Read the model definition and answer for the solid it produces. Units are mm, in the model's axes. A direction names the side the tool comes from. Round coordinates to 2 decimals unless told otherwise and drop trailing zeros. Order: outer loops, then holes, each group sorted by start corner. A loop starts at its lowest first (then second) coordinate and runs counter-clockwise, first axis right, second up. Notation, with made-up numbers: (41, 13) - (54, 13) arc R31 cw to (54, 42) - close; hole circle Ø9 at (-12, -7). An arc over 180 degrees is marked (long way). Answer as a JSON object with one key per item and string values. Group by question number.
Q1. A cutting plane is placed at A-A on x = -3.5. Determine the outline of the cut face in (y, z), and give its area (3 significant figures).
Q2. A cutting plane is placed at D-D on z = -12. Determine the outline of the cut face in (x, y), and give its area (3 significant figures).
Q3. A cutting plane is placed at B-B on z = -65. Determine the outline of the cut face in (x, y).
Q4. The mould has two halves that part along Z. Classify faces 1 (the flat face through (40, 11, -15)), 2 (the cylindrical face through (42.39, 4.27, -66.67)), 3 (the flat face through (10, 63, 24)): pulls with the +Z half, pulls with the -Z half, needs draft (parallel to the pull), parting line crosses it, or undercut.
Q5. A tool of negligible diameter and unlimited length cuts with its end or side. For faces 4 (the flat face through (10, 21, 37)), 5 (the cylindrical face through (-47.61, 4.27, 63.33)), 6 (the flat face through (40, 76, -50)), from which of +Z, -Z, +X, -X, +Y, -Y can it reach the whole face along a straight path? Write none if from no direction.
Q6. Consider line 1 (X direction, y = 10.5, z = 48); line 2 (X direction, y = 1, z = 65); line 3 (Y direction, x = -14.5, z = 24.25). Determine where each line is inside the solid, lowest interval first.
Q7. Given pin 1 Ø5 at (x, z) = (42, 51) entering from +Y; pin 2 Ø12 at (x, y) = (23, 11.5) entering from -Z; pin 3 Ø3 at (x, z) = (-45, 64.5) entering from +Y; pin 4 Ø6 at (x, z) = (14.5, -52) entering from -Y, each flat-ended and moving along its own axis, determine where each tip first touches the part or whether it passes through.
Q8. A cutting plane is placed at C-C on y = 41. Determine the outline of the cut face in (x, z).
```python
from build123d import *

# Parameters (mm, degrees)
SKETCH_1_W               = 110
SKETCH_1_H               = 150
EXTRUDE_1_DEPTH          = 6
SKETCH_2_R               = 6.25
EXTRUDE_2_DEPTH          = 70
SKETCH_3_R               = 1.7
CUT_EXTRUDE_1_DEPTH      = 117.404467268
SKETCH_4_R               = 3.1
CUT_EXTRUDE_2_DEPTH      = 3.5
SKETCH_5_W               = 74.25
SKETCH_5_H               = 6
EXTRUDE_3_DEPTH          = 78
CUT_EXTRUDE_8_DEPTH      = 5
CUT_EXTRUDE_8_DEPTH_BACK = 7
SKETCH_7_R               = 1.6
SKETCH_7_W               = 42
SKETCH_7_H               = 21
SKETCH_10_W              = 12.5
SKETCH_10_H              = 100
EXTRUDE_4_DEPTH          = 5
RIB_3_REACH              = 127.324
SKETCH_8_WALL_W          = 306.935743114
SKETCH_8_WALL_H          = 20
FILLET_5_R               = 2
FILLET_4_R               = 3
CHAMFER_1_SIZE           = 1.5
CHAMFER_2_SIZE           = 0.5


with BuildPart() as part:
    # 草图1 → 凸台-拉伸1 (new body)
    with BuildSketch(Plane(origin=(0, 0, 0), x_dir=(1, 0, 0), z_dir=(0, 1, 0))):
        Rectangle(SKETCH_1_W, SKETCH_1_H)
    extrude(amount=EXTRUDE_1_DEPTH)

    # 草图2 → 凸台-拉伸2 (add)
    with BuildSketch(Plane(origin=(0, 6, 0), x_dir=(1, 0, 0), z_dir=(0, 1, 0))):
        with Locations(Location((-40, 50, 0), (0, 0, 90))):
            Circle(SKETCH_2_R)
        with Locations(Location((40, 50, 0), (0, 0, 90))):
            Circle(SKETCH_2_R)
        with Locations(Location((40, -50, 0), (0, 0, 90))):
            Circle(SKETCH_2_R)
        with Locations(Location((-40, -50, 0), (0, 0, 90))):
            Circle(SKETCH_2_R)
    extrude(amount=EXTRUDE_2_DEPTH)

    # 草图3 → 切除-拉伸1 (cut, through all)
    with BuildSketch(Plane(origin=(0, 6, 0), x_dir=(1, 0, 0), z_dir=(0, 1, 0))):
        with Locations(Location((-45, 65, 0), (0, 0, 270))):
            Circle(SKETCH_3_R)
        with Locations(Location((-45, -65, 0), (0, 0, 90))):
            Circle(SKETCH_3_R)
        with Locations(Location((45, -65, 0), (0, 0, 270))):
            Circle(SKETCH_3_R)
        with Locations(Location((45, 65, 0), (0, 0, 90))):
            Circle(SKETCH_3_R)
    extrude(amount=-CUT_EXTRUDE_1_DEPTH, mode=Mode.SUBTRACT)

    # 草图4 → 切除-拉伸2 (cut)
    with BuildSketch(Plane(origin=(0, 6, 0), x_dir=(1, 0, 0), z_dir=(0, 1, 0))):
        with Locations(Location((-45, 65, 0), (0, 0, 270))):
            Circle(SKETCH_4_R)
        with Locations(Location((45, 65, 0), (0, 0, 90))):
            Circle(SKETCH_4_R)
        with Locations(Location((45, -65, 0), (0, 0, 270))):
            Circle(SKETCH_4_R)
        with Locations(Location((-45, -65, 0), (0, 0, 90))):
            Circle(SKETCH_4_R)
    extrude(amount=-CUT_EXTRUDE_2_DEPTH, mode=Mode.SUBTRACT)

    # 草图5 → 凸台-拉伸3 (add)
    with BuildSketch(Plane(origin=(0, 6, 0), x_dir=(1, 0, 0), z_dir=(0, 1, 0))):
        with Locations((9.125, -24)):
            Rectangle(SKETCH_5_W, SKETCH_5_H)
    extrude(amount=EXTRUDE_3_DEPTH)

    # 草图7 → 切除-拉伸8 (cut, two sides: drawn at the far end of the back side and taken through both)
    with BuildSketch(Plane.XY.offset(27).offset(-CUT_EXTRUDE_8_DEPTH_BACK)):
        with Locations(Location((-14.5, 69, 0), (0, 0, 180))):
            Circle(SKETCH_7_R)
        with Locations(Location((-14.5, 79, 0), (0, 0, 180))):
            Circle(SKETCH_7_R)
        with Locations(Location((34.5, 69, 0), (0, 0, 180))):
            Circle(SKETCH_7_R)
        with Locations(Location((34.5, 79, 0), (0, 0, 180))):
            Circle(SKETCH_7_R)
        with Locations((10, 73.5)):
            Rectangle(SKETCH_7_W, SKETCH_7_H)
    extrude(amount=CUT_EXTRUDE_8_DEPTH + CUT_EXTRUDE_8_DEPTH_BACK, mode=Mode.SUBTRACT)

    # 草图10 → 凸台-拉伸4 (add)
    with BuildSketch(Plane(origin=(0, 6, 0), x_dir=(1, 0, 0), z_dir=(0, 1, 0))):
        Polygon((-33.75, -50), (-33.75, -27), (-28, -27), (-28, -21), (-33.75, -21), (-33.75, 50), (-46.25, 50), (-46.25, -50), align=None)
        with Locations((40, 0)):
            Rectangle(SKETCH_10_W, SKETCH_10_H)
    extrude(amount=EXTRUDE_4_DEPTH)

    # 草图8 wall → 筋3 (add, up to next)
    with BuildSketch(Plane(origin=(0, 26.75, 44.5), x_dir=(0, -0.764433319597, 0.64470279966), z_dir=(0, -0.64470279966, -0.764433319597)), mode=Mode.PRIVATE) as rib_3_sk1:
        Rectangle(SKETCH_8_WALL_W, SKETCH_8_WALL_H)
    rib_3_tool1 = extrude(rib_3_sk1.sketch, amount=RIB_3_REACH, mode=Mode.PRIVATE) - part.part
    add(rib_3_tool1.solids().sort_by_distance((0, 26.75, 44.5))[0])

    # 圆角5
    fillet_5_edges = [part.edges().sort_by_distance(p)[0] for p in [
        (35.580582618, 6, -54.419417382),
        (-44.419417382, 6, -54.419417382),
        (0, 6, 21),
        (40, 6, 56.25),
        (-46.25, 6, 0),
        (-33.75, 6, 38.5),
        (-33.75, 6, -14.5),
        (-40, 6, 56.25),
        (33.75, 6, 38.5),
        (33.75, 6, -14.5),
        (21.875, 6, 27),
        (0, 6, 62),
        (-21.875, 6, 27),
        (46.25, 6, 0),
    ]]
    fillet(fillet_5_edges, radius=FILLET_5_R)

    # 圆角4
    fillet_4_edges = [part.edges().sort_by_distance(p)[0] for p in [
        (-11, 63, 24),
        (31, 63, 24),
        (0, 6, 75),
        (-55, 6, 0),
        (0, 6, -75),
        (-28, 84, 24),
        (46.25, 84, 24),
        (55, 6, 0),
        (31, 84, 24),
        (-11, 84, 24),
    ]]
    fillet(fillet_4_edges, radius=FILLET_4_R)

    # 倒角1
    chamfer_1_edges = [part.edges().sort_by_distance(p)[0] for p in [
        (-40, 76, 56.25),
        (40, 76, 56.25),
        (40, 76, -43.75),
        (-40, 76, -43.75),
    ]]
    chamfer(chamfer_1_edges, length=CHAMFER_1_SIZE)

    # 倒角2
    chamfer_2_edges = [part.edges().sort_by_distance(p)[0] for p in [
        (36.1, 79, 27),
        (36.1, 79, 21),
        (36.1, 69, 27),
        (36.1, 69, 21),
        (-12.9, 79, 27),
        (-12.9, 79, 21),
        (-12.9, 69, 27),
        (-12.9, 69, 21),
    ]]
    chamfer(chamfer_2_edges, length=CHAMFER_2_SIZE)


solid = part.part
```
Result set:
{
 "1": {"outline": "(0, -75) - (3, -75) arc R3 ccw to (6, -72) - (6, 19) arc R2 cw to (8, 21) - (63, 21) - (63, 27) - (47.5, 27) - (6.71, 61.4) arc R2 cw to (6, 62.93) - (6, 72) arc R3 ccw to (3, 75) - (0, 75) - close", "area": "1,970 mm²"},
 "2": {"outline": "(-55, 0) - (55, 0) - (55, 3) arc R3 ccw to (52, 6) - (48.25, 6) arc R2 cw to (46.25, 8) - (46.25, 11) - (33.75, 11) - (33.75, 8) arc R2 cw to (31.75, 6) - (-31.75, 6) arc R2 cw to (-33.75, 8) - (-33.75, 11) - (-46.25, 11) - (-46.25, 8) arc R2 cw to (-48.25, 6) - (-52, 6) arc R3 ccw to (-55, 3) - close", "area": "785 mm²"},
 "3": {"outline": "(-55, 0) - (-46.7, 0) - (-46.7, 2.5) - (-48.1, 2.5) - (-48.1, 6) - (-52, 6) arc R3 ccw to (-55, 3) - close; (-43.3, 0) - (43.3, 0) - (43.3, 2.5) - (41.9, 2.5) - (41.9, 6) - (-41.9, 6) - (-41.9, 2.5) - (-43.3, 2.5) - close; (46.7, 0) - (55, 0) - (55, 3) arc R3 ccw to (52, 6) - (48.1, 6) - (48.1, 2.5) - (46.7, 2.5) - close"},
 "4": {"face 1": "undercut", "face 2": "undercut", "face 3": "needs draft"},
 "5": {"face 4": "+Z, +Y", "face 5": "+Y", "face 6": "-Z, +X, -X, +Y"},
 "6": {"line 1": "x = -46.25 to -33.75, -10 to 10, 33.75 to 46.25", "line 2": "x = -55 to -46.7, -43.3 to 43.3, 46.7 to 55", "line 3": "y = 0 to 67.4, 70.6 to 77.4, 80.6 to 84"},
 "7": {"pin 1": "stops at y = 76", "pin 2": "stops at z = -73.66", "pin 3": "stops at y = 2.5", "pin 4": "stops at y = 0"},
 "8": {"outline": "circle Ø12.5 at (-40, -50); circle Ø12.5 at (-40, 50); (-28, 21) - (46.25, 21) - (46.25, 27) - (10, 27) - (10, 32.48) - (-10, 32.48) - (-10, 27) - (-28, 27) - close; circle Ø12.5 at (40, -50); circle Ø12.5 at (40, 50)"}
}
